Work out the finished part from the listing and answer in its coordinate system (mm). A direction names the side the tool comes from. Coordinates: 2 decimals unless noted, no trailing zeros. Write each loop counter-clockwise with the first axis right and the second up, starting at its lowest first coordinate (ties: lowest second). Pieces come first, ordered by that corner, then holes. Notation, with made-up numbers: (71, 55) - (82, 55) arc R32 cw to (82, 85) - close; hole circle Ø4 at (7.25, -0.75). An arc over 180 degrees is marked (long way). One line per item, written item: value.
```python
from build123d import *

# Parameters (mm, degrees)
SKETCH1_W           = 30.48
SKETCH1_H           = 40.64
BOSS_EXTRUDE1_DEPTH = 20.32
SKETCH2_W           = 39.2176
SKETCH2_H           = 39.2176
CUT_EXTRUDE1_DEPTH  = 29.0576
SKETCH3_R           = 1.27
CUT_EXTRUDE2_DEPTH  = 2.4224
SKETCH4_R           = 3.81
BOSS_EXTRUDE2_DEPTH = 19.05
FILLET1_R           = 2.54


with BuildPart() as part:
    # Sketch1 → Boss-Extrude1 (new body, symmetric)
    with BuildSketch(Plane(origin=(0, 0, 0), x_dir=(1, 0, 0), z_dir=(0, 1, 0))):
        Rectangle(SKETCH1_W, SKETCH1_H)
    extrude(amount=BOSS_EXTRUDE1_DEPTH, both=True)

    # Sketch2 → Cut-Extrude1 (cut)
    with BuildSketch(Plane(origin=(15.24, 0, 0), x_dir=(0, 0, -1), z_dir=(1, 0, 0))):
        with Locations((0.7112, 0.7112)):
            Rectangle(SKETCH2_W, SKETCH2_H)
    extrude(amount=-CUT_EXTRUDE1_DEPTH, mode=Mode.SUBTRACT)

    # Sketch3 → Cut-Extrude2 (cut, through all)
    with BuildSketch(Plane(origin=(0, -18.8976, 0), x_dir=(1, 0, 0), z_dir=(0, 1, 0))):
        with Locations((-5.08, -7.62)):
            Circle(SKETCH3_R)
        with Locations((7.62, -7.62)):
            Circle(SKETCH3_R)
        with Locations((0, 7.62)):
            Circle(SKETCH3_R)
    extrude(amount=-CUT_EXTRUDE2_DEPTH, mode=Mode.SUBTRACT)

    # Sketch4 → Boss-Extrude2 (add)
    with BuildSketch(Plane.ZY.offset(15.24)):
        with Locations((0, 1.27)):
            Circle(SKETCH4_R)
    extrude(amount=BOSS_EXTRUDE2_DEPTH)

    # Sketch5 → Revolve1 (revolve)
    with BuildSketch(Plane.XY):
        Polygon((-30.48, 5.08), (-30.48, 10.16), (-28.8036, 10.16), (-28.8036, 7.112), (-21.8186, 7.112), (-21.8186, 10.16), (-20.1422, 10.16), (-20.1422, 5.08), align=None)
    revolve(axis=Axis((-34.29, 1.27, 0), (1, 0, 0)))

    # Fillet1
    fillet1_edges = [part.edges().sort_by_distance(p)[0] for p in [
        (-34.29, 1.27, -3.81),
    ]]
    fillet(fillet1_edges, radius=FILLET1_R)


solid = part.part
```
Item 1: Section B-B, the plane y = 9 is taken. Determine the outline of the cut face in (x, z).
Evaluation:
outline: (-30.48, -4.39) - (-28.8, -4.39) - (-28.8, 4.39) - (-30.48, 4.39) - close; (-21.82, -4.39) - (-20.14, -4.39) - (-20.14, 4.39) - (-21.82, 4.39) - close; (-15.24, -20.32) - (-13.82, -20.32) - (-13.82, 18.9) - (15.24, 18.9) - (15.24, 20.32) - (-15.24, 20.32) - close
Item 2: Section D-D, the plane z = 5 is taken. Determine the outline of the cut face in (x, y), then the cut area to 3 significant figures.
Evaluation:
outline: (-30.48, -6.08) - (-28.8, -6.08) - (-28.8, -1.75) - (-21.82, -1.75) - (-21.82, -6.08) - (-20.14, -6.08) - (-20.14, 8.62) - (-21.82, 8.62) - (-21.82, 4.29) - (-28.8, 4.29) - (-28.8, 8.62) - (-30.48, 8.62) - close; (-15.24, -20.32) - (15.24, -20.32) - (15.24, -18.9) - (-13.82, -18.9) - (-13.82, 20.32) - (-15.24, 20.32) - close
area: 191 mm2
Item 3: Given pin 1 (1.5 mm diameter, centred on x = 7.62, z = 7.62, fed in from -Y); pin 2 (6 mm diameter, centred on y = 14.5, z = 13.5, fed in from -X); pin 3 (5.5 mm diameter, centred on y = 3, z = -3.5, fed in from +X); pin 4 (9 mm diameter, centred on y = 5.5, z = -1, fed in from -X), each flat-ended and moving along its own axis, determine where each tip first touches the part or whether it passes through.
Evaluation:
pin 1: passes through
pin 2: stops at x = -15.24
pin 3: stops at x = -13.82
pin 4: stops at x = -34.29
Item 4: Consider probe 1 along X at (y, z) = (-19.3, 7.62); probe 2 along Z at (x, y) = (-5.08, -19.4); probe 3 along Z at (x, y) = (0, -19). Determine where each line is inside the solid, lowest interval first.
Evaluation:
probe 1: x = -15.24 to -6.35, -3.81 to 6.35, 8.89 to 15.24
probe 2: z = -20.32 to 6.35, 8.89 to 20.32
probe 3: z = -20.32 to -8.89, -6.35 to 20.32
Item 5: Determine the mould class of faces 4 (the face through (-25.26, -3.37, -3.55)), 5 (the face through (-17.657, 5.048, -0.496)), 6 (the face through (1, 0, 18.898)), 7 (the face through (-34.29, 1, 0)) for opening direction X: +X half, -X half, draft (parallel to the pull), parting line (faces both ways), or undercut.
Evaluation:
face 4: undercut
face 5: undercut
face 6: draft
face 7: -X half
Item 6: Section C-C, the plane z = -7.62 is taken. Determine the outline of the cut face in (x, y), then the cut area to 3 significant figures.
Evaluation:
outline: (-30.48, -3.31) - (-28.8, -3.31) - (-28.8, 5.85) - (-30.48, 5.85) - close; (-21.82, -3.31) - (-20.14, -3.31) - (-20.14, 5.85) - (-21.82, 5.85) - close; (-15.24, -20.32) - (-1.27, -20.32) - (-1.27, -18.9) - (-13.82, -18.9) - (-13.82, 20.32) - (-15.24, 20.32) - close; (1.27, -20.32) - (15.24, -20.32) - (15.24, -18.9) - (1.27, -18.9) - close
area: 126 mm2
Item 7: Which of the six approach directions +Z, -Z, +X, -X, +Y, -Y give full straight-line access (tool end or side, diameter ignored) to faces 1 (the face through (-28.804, 7, -2)), 2 (the face through (-13.818, 1, 0)), 3 (the face through (-31.106, 5.048, -0.496))?
Evaluation:
face 1: none
face 2: -Z, +X, +Y
face 3: -X
Item 8: Section A-A, the plane x = 0 is taken. Determine the outline of the cut face in (y, z), then the cut area to 3 significant figures.
Evaluation:
outline: (-20.32, -20.32) - (-18.9, -20.32) - (-18.9, -8.89) - (-20.32, -8.89) - close; (-20.32, -6.35) - (-18.9, -6.35) - (-18.9, 18.9) - (20.32, 18.9) - (20.32, 20.32) - (-20.32, 20.32) - close
area: 110 mm2
